Verification items for the finished model (mm, model axes). Face numbers are marked on the shaded views. A direction names the side the tool comes from. Round coordinates to 2 decimals unless told otherwise and drop trailing zeros. Write each loop counter-clockwise with the first axis right and the second up, starting at its lowest first coordinate (ties: lowest second). Pieces come first, ordered by that corner, then holes. Notation, with made-up numbers: (82, 58) - (128, 58) arc R28 ccw to (128, 88) - close; hole circle Ø6 at (37, -11). An arc over 180 degrees is marked (long way). Answer as a JSON object with one key per item and string values. Group by question number.
1) Section check B-B (y = 5). Enter the section's corners in (x, z).
2) Thickness scan on line 1 (Y direction, x = 17, z = 39); line 2 (Z direction, x = 68.5, y = 11.75); line 3 (Y direction, x = 93.5, z = -34.5). Record the ranges inside material, lowest first.
3) Section check C-C (x = 57). Enter the section's corners in (y, z).
4) Section check D-D (z = -38.5). Enter the section's corners in (x, y), then the cut area to 3 significant figures.
5) Go/stop test with a flat-tipped pin: pin 1 Ø3 at (x, z) = (20, -23.5) entering from -Y. Record where the tip stops, or that it passes through.
6) Set-up check for the marked faces 1 and 2: record each of +Z, -Z, +X, -X, +Y, -Y from which the full face is reachable in a straight line by a thin tool's end or side.
7) Mould release check, pull along Y, two halves, no side actions. Record for the marked faces 3, 4, 5 and 6: +Y half, -Y half, draft (parallel to the pull), parting line (faces both ways), or undercut.
8) Section check A-A (z = 37). Enter the section's corners in (x, y).
```python
from build123d import *

# Parameters (mm, degrees)
SALIENTE_EXTRUIR1_DEPTH = 100
SALIENTE_EXTRUIR2_DEPTH = 100


with BuildPart() as part:
    # Croquis1 → Saliente-Extruir1 (new body)
    with BuildSketch(Plane(origin=(0, 0, 0), x_dir=(0, 0, -1), z_dir=(1, 0, 0))):
        Polygon((-30, 3.5), (-40, 13.5), (40, 13.5), (30, 3.5), (50, 3.5), (50, 18.770945102), (-50, 18.770945102), (-50, 3.5), align=None)
    extrude(amount=SALIENTE_EXTRUIR1_DEPTH)

    # Croquis2 → Saliente-Extruir2 (add)
    with BuildSketch(Plane(origin=(0, 0, -50), x_dir=(-1, 0, 0), z_dir=(0, 0, -1))):
        Polygon((-80, 18.770945102), (-90, 28.770945102), (-10, 28.770945102), (-20, 18.770945102), align=None)
    extrude(amount=-SALIENTE_EXTRUIR2_DEPTH)


solid = part.part
```
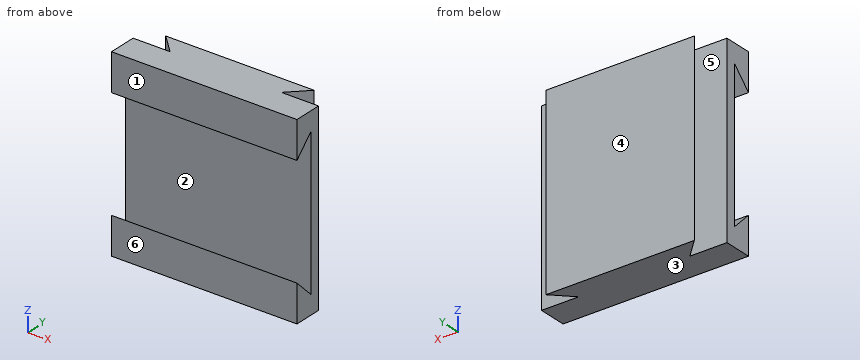
Returned:
{
 "1": {"outline": "(0, -50) - (100, -50) - (100, -31.5) - (0, -31.5) - close; (0, 31.5) - (100, 31.5) - (100, 50) - (0, 50) - close"},
 "2": {"line 1": "3.5 to 12.5, 13.5 to 18.77, 21.77 to 28.77", "line 2": "-50 to -38.25, 38.25 to 50", "line 3": "3.5 to 8, 13.5 to 18.77"},
 "3": {"outline": "(3.5, -50) - (28.77, -50) - (28.77, 50) - (3.5, 50) - (3.5, 30) - (13.5, 40) - (13.5, -40) - (3.5, -30) - close"},
 "4": {"outline": "(0, 3.5) - (100, 3.5) - (100, 12) - (0, 12) - close; (0, 13.5) - (100, 13.5) - (100, 18.77) - (80, 18.77) - (90, 28.77) - (10, 28.77) - (20, 18.77) - (0, 18.77) - close", "area": "2,080 mm2"},
 "5": {"pin 1": "y = 13.5"},
 "6": {"face 1": "+Z, -Z, +X, -X, -Y", "face 2": "+X, -X"},
 "7": {"face 3": "draft", "face 4": "+Y half", "face 5": "undercut", "face 6": "-Y half"},
 "8": {"outline": "(0, 3.5) - (100, 3.5) - (100, 10.5) - (0, 10.5) - close; (0, 13.5) - (100, 13.5) - (100, 18.77) - (80, 18.77) - (90, 28.77) - (10, 28.77) - (20, 18.77) - (0, 18.77) - close"}
}
